Build history of the part. All positions in model axes, mm. A direction names the side the tool comes from. Give positions to 0.01 mm unless a question says otherwise; leave off trailing zeros. Order: outer loops, then holes, each group sorted by start corner. A loop starts at its lowest first (then second) coordinate and runs counter-clockwise, first axis right, second up. Notation, with made-up numbers: (-25, 88) - (-9, 88) arc R35 cw to (-9, 123) - close; hole circle Ø4 at (79, 48). An arc over 180 degrees is marked (long way). Write each question's results on one line, items separated by ' | '. Start each with the question number.
1) Cut at D-D on z = -7.5. List the corners of the cut face in (x, y), plus the area to 3 significant figures.
2) Cut at A-A on x = -16. List the corners of the cut face in (y, z), plus the area to 3 significant figures.
3) Drill centre lines: line 1 along Z through (x, y) = (-16, -6); line 2 along Z through (x, y) = (12, -4); line 3 along Y through (x, z) = (5.5, -34). Where is each one in solid material? Low to high. Write a range as from..to.
4) Tool access for faces 5 (the face through (24, 17, -12)), 6 (the face through (12, 17, -24)), 7 (the face through (12, -3, -40)): list every direction of +Z, -Z, +X, -X, +Y, -Y with a clear straight run to the whole face (end or side of a thin tool).
5) Cut at C-C on x = 12. List the corners of the cut face in (y, z), plus the area to 3 significant figures.
6) Two-plate mould, pull along X, no slides. Class faces 1 (the face through (12, -5, 20.5)), 2 (the face through (11.46, -6.55, -42.44)), 3 (the face through (0, 17, -12)), 4 (the face through (44.5, -5, -12)): +X half, -X half, draft (parallel to the pull), parting line (faces both ways), or undercut.
7) Drop flat-ended pins along their axis: pin 1 Ø1.5 at (y, z) = (30, -25) entering from -X; pin 2 Ø6 at (x, y) = (19.5, 10) entering from -Z; pin 3 Ø6.5 at (x, z) = (-16, 16) entering from +Y; pin 4 Ø7 at (y, z) = (13, -15) entering from -X. Give the stop position or say it passes through.
8) Cut at B-B on z = -40. List the corners of the cut face in (x, y), plus the area to 3 significant figures.
from build123d import *

# Parameters (mm, degrees)
SKETCH1_W           = 24
SKETCH1_H           = 24
BOSS_EXTRUDE1_DEPTH = 35
SKETCH2_W           = 65
SKETCH2_H           = 65
SKETCH2_R           = 2
BOSS_EXTRUDE2_DEPTH = 10
SKETCH3_R           = 2.5
CUT_EXTRUDE1_DEPTH  = 7


with BuildPart() as part:
    # Sketch1 → Boss-Extrude1 (new body)
    with BuildSketch(Plane(origin=(0, 0, 0), x_dir=(1, 0, 0), z_dir=(0, 1, 0))):
        with Locations((12, 12)):
            Rectangle(SKETCH1_W, SKETCH1_H)
    extrude(amount=BOSS_EXTRUDE1_DEPTH)

    # Sketch2 → Boss-Extrude2 (add)
    with BuildSketch(Plane.XZ):
        with Locations((12, -12)):
            Rectangle(SKETCH2_W, SKETCH2_H)
        with Locations((-16, 16)):
            Circle(SKETCH2_R, mode=Mode.SUBTRACT)
        with Locations((-16, -40)):
            Circle(SKETCH2_R, mode=Mode.SUBTRACT)
        with Locations((40, 16)):
            Circle(SKETCH2_R, mode=Mode.SUBTRACT)
        with Locations((40, -40)):
            Circle(SKETCH2_R, mode=Mode.SUBTRACT)
    extrude(amount=BOSS_EXTRUDE2_DEPTH)

    # Sketch3 → Cut-Extrude1 (cut)
    with BuildSketch(Plane.XZ.offset(10)):
        with Locations((12, 16)):
            Circle(SKETCH3_R)
        with Locations((12, -40)):
            Circle(SKETCH3_R)
    extrude(amount=-CUT_EXTRUDE1_DEPTH, mode=Mode.SUBTRACT)


solid = part.part
Results:
1) outline: (-20.5, -10) - (44.5, -10) - (44.5, 0) - (24, 0) - (24, 35) - (0, 35) - (0, 0) - (-20.5, 0) - close | area: 1,490 mm^2
2) outline: (-10, -44.5) - (0, -44.5) - (0, -42) - (-10, -42) - close; (-10, -38) - (0, -38) - (0, 14) - (-10, 14) - close; (-10, 18) - (0, 18) - (0, 20.5) - (-10, 20.5) - close | area: 570 mm^2
3) line 1: -44.5..-42, -38..14, 18..20.5 | line 2: -44.5..-42.5, -37.5..13.5, 18.5..20.5 | line 3: -10..0
4) face 5: +Z, -Z, +X, +Y | face 6: -Z, +X, -X, +Y | face 7: -Y
5) outline: (-10, -44.5) - (0, -44.5) - (0, -24) - (35, -24) - (35, 0) - (0, 0) - (0, 20.5) - (-10, 20.5) - (-10, 18.5) - (-3, 18.5) - (-3, 13.5) - (-10, 13.5) - (-10, -37.5) - (-3, -37.5) - (-3, -42.5) - (-10, -42.5) - close | area: 1,420 mm^2
6) face 1: draft | face 2: undercut | face 3: -X half | face 4: +X half
7) pin 1: through | pin 2: z = -24 | pin 3: y = 0 | pin 4: x = 0
8) outline: (-20.5, -10) - (-18, -10) - (-18, 0) - (-20.5, 0) - close; (-14, -10) - (9.5, -10) - (9.5, -3) - (14.5, -3) - (14.5, -10) - (38, -10) - (38, 0) - (-14, 0) - close; (42, -10) - (44.5, -10) - (44.5, 0) - (42, 0) - close | area: 535 mm^2
